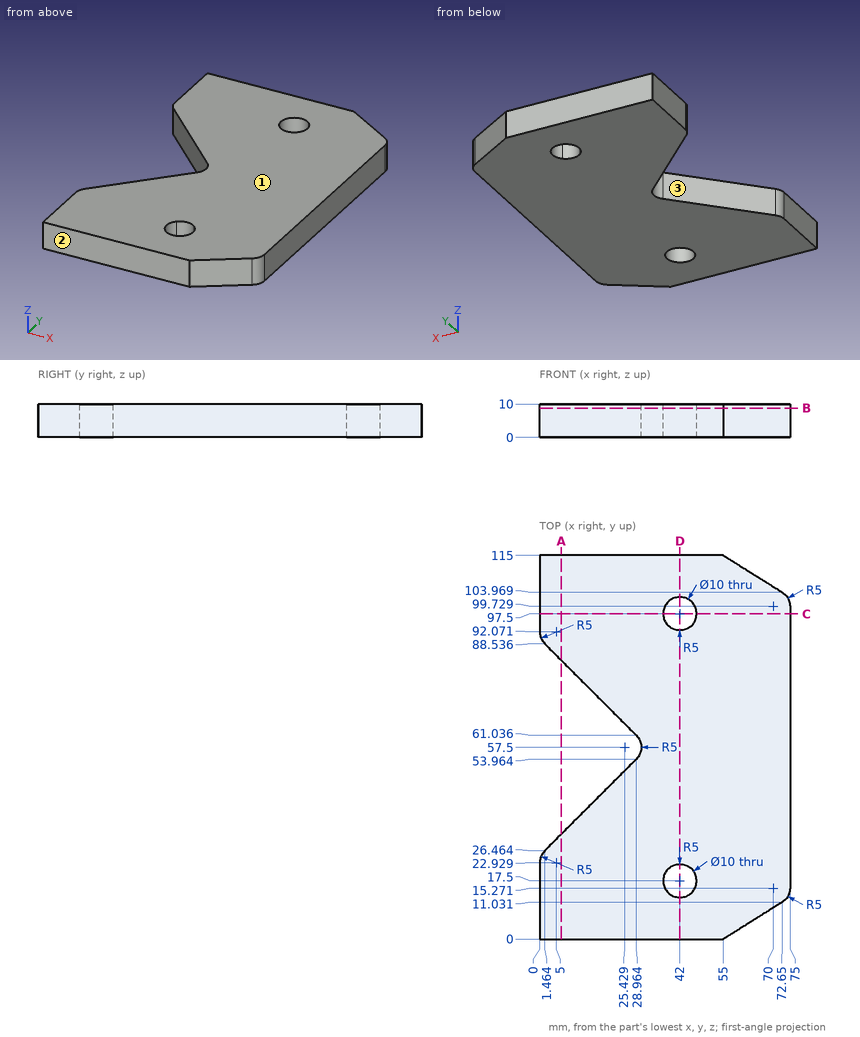
Design review of the part shown in the three views and the two pictorial views. Dimensions are in mm from the part's minimum x, y and z. Round coordinates to 2 decimals unless told otherwise and drop trailing zeros. Order: outer loops, then holes, each group sorted by start corner. A loop starts at its lowest first (then second) coordinate and runs counter-clockwise, first axis right, second up. Notation, with made-up numbers: M -24,81 L -7,81 A14 ccw -7,100 Z; hole C 87.5,36.5 d7. An arc over 180 degrees is marked long. Put each result on its own line as item: value.
Q1. To check wall thickness, follow line 1 (X direction, y = 17.5, z = 6.75); line 2 (Y direction, x = 44.5, z = 9); line 3 (Y direction, x = 46, z = 8). State the ranges of each line that lie inside material, in increasing order.
Reported:
line 1: 0 to 37, 47 to 75
line 2: 0 to 13.17, 21.83 to 93.17, 101.83 to 115
line 3: 0 to 14.5, 20.5 to 94.5, 100.5 to 115
Q2. Consider section B-B (z = 8.75). State how many separate pieces and enclosed holes the cut face has, and give its area (3 significant figures).
Reported:
separate pieces: 1
enclosed holes: 2
area: 7,160 mm²
Q3. Consider section A-A (x = 6.5). State the section outline as (y, z) points, and give its area (3 significant figures).
Reported:
outline: M 0,0 L 31.5,0 L 31.5,10 L 0,10 Z; M 83.5,0 L 115,0 L 115,10 L 83.5,10 Z
area: 630 mm²
Q4. Consider section D-D (x = 42). State the section outline as (y, z) points.
Reported:
outline: M 0,0 L 12.5,0 L 12.5,10 L 0,10 Z; M 22.5,0 L 92.5,0 L 92.5,10 L 22.5,10 Z; M 102.5,0 L 115,0 L 115,10 L 102.5,10 Z
Q5. Draft analysis for pull direction Y (two halves, no side actions). For the marked faces 1, 2 and 3, state which applies: released by +Y, released by -Y, zero draft, split by the parting line, or undercut.
Reported:
face 1: zero draft
face 2: released by -Y
face 3: undercut
Q6. Insertion check: pin 1 Ø8 at (x, y) = (42, 17.5) entering from -Z; pin 2 Ø6 at (y, z) = (57.5, 6.5) entering from -X. Each pin has a flat end and moves straight along its axis. Give the tip position at first contact, or say it passes through.
Reported:
pin 1: through
pin 2: x = 29.43
Q7. Consider section C-C (y = 97.5). State the section outline as (x, z) points, and give its area (3 significant figures).
Reported:
outline: M 0,0 L 37,0 L 37,10 L 0,10 Z; M 47,0 L 75,0 L 75,10 L 47,10 Z
area: 650 mm²
